Verification items for the finished model (mm, model axes). A direction names the side the tool comes from. Give positions to 0.01 mm unless a question says otherwise; leave off trailing zeros. Order: outer loops, then holes, each group sorted by start corner. A loop starts at its lowest first (then second) coordinate and runs counter-clockwise, first axis right, second up. Notation, with made-up numbers: (10, 39.5) -> (37, 39.5) arc R18 cw to (37, 73.5) -> close; hole circle Ø6 at (11, -4.5). An arc over 180 degrees is marked (long way). Return JSON: item names as keys, results as strings. Group by question number.
(1) Tool access check on faces 1 (the face through (0, 3, 4.72)), 2 (the face through (1.43, -2.75, 9.75)), 3 (the face through (-0.759, -3.417, 4.93)), 4 (the face through (1.43, -2.75, 0.25)). Record the directions out of +Z, -Z, +X, -X, +Y, -Y that give a thin tool (end or side, any length) a straight path to the whole face; none if there is none.
(2) Thickness scan on line 1 along Y through (x, z) = (0, 2.5); line 2 along Y through (x, z) = (0, 0.3); line 3 along Z through (x, y) = (1.5, 3). Record the ranges inside material, lowest first.
(3) Cross-section at A-A on y = 0. Enter the section's corners in (x, z), then the cut area to 3 significant figures.
(4) Depth check by flat-ended pin: pin 1 Ø1.7 at (x, y) = (0, 2) entering from +Z; pin 2 Ø1.9 at (x, y) = (-1.5, 0) entering from -Z. Enter the tip coordinate at first touch or a pass-through.
(5) Cross-section at B-B on x = 0. Enter the section's corners in (y, z).
(6) Release check for a two-part mould opening along Z. For faces 5 (the face through (0, 3, 5.28)), 6 (the face through (2, -2, 0.5)), 7 (the face through (-2.398, 0.106, 5.063)), 8 (the face through (2, -2, 9.5)) record: pulls with the +Z half, pulls with the -Z half, needs draft (parallel to the pull), parting line crosses it, or undercut.
(7) Cross-section at C-C on z = 8.5. Enter the section's corners in (x, y), then the cut area to 3 significant figures.
(8) Cross-section at D-D on y = 2.25. Enter the section's corners in (x, z).
from build123d import *

# Parameters (mm, degrees)
SKETCH1_R           = 3.5
BOSS_EXTRUDE1_DEPTH = 10
SKETCH3_R           = 2.4
CUT_EXTRUDE1_DEPTH  = 12.157956802
SKETCH4_R           = 3.1
CUT_EXTRUDE2_DEPTH  = 0.5
WRAP1_SECTION_W     = 1
WRAP1_SECTION_H     = 0.5606788
WRAP1_ANGLE         = 114.591559026


with BuildPart() as part:
    # Sketch1 → Boss-Extrude1 (new body)
    with BuildSketch(Plane.XY):
        Circle(SKETCH1_R)
    extrude(amount=BOSS_EXTRUDE1_DEPTH)

    # Sketch3 → Cut-Extrude1 (cut, through all)
    with BuildSketch(Plane.XY.offset(10)):
        Circle(SKETCH3_R)
    extrude(amount=-CUT_EXTRUDE1_DEPTH, mode=Mode.SUBTRACT)

    # Sketch4 → Cut-Extrude2 (cut)
    with BuildSketch(Plane.XY.offset(10)):
        Circle(SKETCH4_R)
    cut_extrude2 = extrude(amount=-CUT_EXTRUDE2_DEPTH, mode=Mode.SUBTRACT)

    # Mirror1: Cut-Extrude2 across plane
    add(cut_extrude2.mirror(Plane.XY.offset(5)), mode=Mode.SUBTRACT)

    # Wrap1 section (on wrap section) → Wrap1 (revolve, cut)
    with BuildSketch(Plane(origin=(0, 0, 0), x_dir=(-0.8414709848078967, 0.5403023058681393, 0), z_dir=(-0.5403023058681393, -0.8414709848078967, 0))):
        with Locations((3, -5)):
            Rectangle(WRAP1_SECTION_W, WRAP1_SECTION_H)
    revolve(axis=Axis((0, 0, 0), (0, 0, -1)), revolution_arc=WRAP1_ANGLE, mode=Mode.SUBTRACT)


solid = part.part
Verdict:
{
 "1": {"face 1": "+Y", "face 2": "+Z", "face 3": "+Z, -Z", "face 4": "-Z"},
 "2": {"line 1": "-3.5 to -2.4, 2.4 to 3.5", "line 2": "-3.5 to -3.1, 3.1 to 3.5", "line 3": "0 to 4.72, 5.28 to 10"},
 "3": {"outline": "(-3.5, 0) -> (-3.1, 0) -> (-3.1, 0.5) -> (-2.4, 0.5) -> (-2.4, 9.5) -> (-3.1, 9.5) -> (-3.1, 10) -> (-3.5, 10) -> close; (2.4, 0.5) -> (3.1, 0.5) -> (3.1, 0) -> (3.5, 0) -> (3.5, 10) -> (3.1, 10) -> (3.1, 9.5) -> (2.4, 9.5) -> close", "area": "20.6 mm²"},
 "4": {"pin 1": "z = 9.5", "pin 2": "z = 0.5"},
 "5": {"outline": "(-3.5, 0) -> (-3.1, 0) -> (-3.1, 0.5) -> (-2.4, 0.5) -> (-2.4, 9.5) -> (-3.1, 9.5) -> (-3.1, 10) -> (-3.5, 10) -> close; (2.4, 0.5) -> (3.1, 0.5) -> (3.1, 0) -> (3.5, 0) -> (3.5, 4.72) -> (2.5, 4.72) -> (2.5, 5.28) -> (3.5, 5.28) -> (3.5, 10) -> (3.1, 10) -> (3.1, 9.5) -> (2.4, 9.5) -> close"},
 "6": {"face 5": "undercut", "face 6": "pulls with the -Z half", "face 7": "needs draft", "face 8": "pulls with the +Z half"},
 "7": {"outline": "circle Ø7 at (0, 0); hole circle Ø4.8 at (0, 0)", "area": "20.4 mm²"},
 "8": {"outline": "(-2.68, 0) -> (-2.13, 0) -> (-2.13, 0.5) -> (-0.84, 0.5) -> (-0.84, 9.5) -> (-2.13, 9.5) -> (-2.13, 10) -> (-2.68, 10) -> (-2.68, 5.28) -> (-1.09, 5.28) -> (-1.09, 4.72) -> (-2.68, 4.72) -> close; (0.84, 0.5) -> (2.13, 0.5) -> (2.13, 0) -> (2.68, 0) -> (2.68, 4.72) -> (1.09, 4.72) -> (1.09, 5.28) -> (2.68, 5.28) -> (2.68, 10) -> (2.13, 10) -> (2.13, 9.5) -> (0.84, 9.5) -> close"}
}
